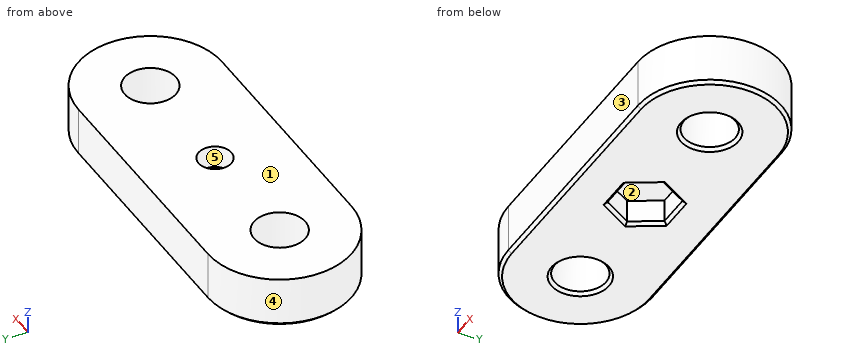
from build123d import *

# Parameters (mm, degrees)
SKETCH_R        = 2.5
SKETCH_R_2      = 1.6
PAD_DEPTH       = 5
POCKET_DEPTH    = 2.5
SKETCH002_R     = 1.6
PAD001_DEPTH    = 0.3
CHAMFER_SIZE    = 0.3
CHAMFER001_SIZE = 0.3


with BuildPart() as part:
    # Sketch → Pad (new body)
    with BuildSketch(Plane.XY):
        with BuildLine():
            ThreePointArc((-11.575, 7), (-18.575, 0), (-11.575, -7))
            Line((-11.575, -7), (11.575, -7))
            ThreePointArc((11.575, -7), (18.575, 0), (11.575, 7))
            Line((-11.575, 7), (11.575, 7))
        make_face()
        with Locations((-11.575, 0)):
            Circle(SKETCH_R, mode=Mode.SUBTRACT)
        with Locations((11.575, 0)):
            Circle(SKETCH_R, mode=Mode.SUBTRACT)
        Circle(SKETCH_R_2, mode=Mode.SUBTRACT)
    extrude(amount=PAD_DEPTH)

    # Sketch001 → Pocket (cut)
    with BuildSketch(Plane(origin=(0, 0, 0), x_dir=(1, 0, 0), z_dir=(0, 0, -1))):
        Polygon((1.602147, 2.775), (-1.602147, 2.775), (-3.204294, 0), (-1.602147, -2.775), (1.602147, -2.775), (3.204294, 0), align=None)
    extrude(amount=-POCKET_DEPTH, mode=Mode.SUBTRACT)

    # Sketch002 → Pad001 (new body)
    with BuildSketch(Plane(origin=(0, 0, 2.5), x_dir=(1, 0, 0), z_dir=(0, 0, -1))):
        Circle(SKETCH002_R)
    extrude(amount=-PAD001_DEPTH)

    # Chamfer
    chamfer_edges = [part.edges().sort_by_distance(p)[0] for p in [
        (-14.075, 0, 0),
        (9.075, 0, 0),
        (2.40322, -1.3875, 0),
        (0, -2.775, 0),
        (-2.40322, -1.3875, 0),
        (-2.40322, 1.3875, 0),
        (0, 2.775, 0),
        (2.40322, 1.3875, 0),
    ]]
    chamfer(chamfer_edges, length=CHAMFER_SIZE)

    # Chamfer001
    chamfer001_edges = [part.edges().sort_by_distance(p)[0] for p in [
        (0, 7, 0),
    ]]
    chamfer(chamfer001_edges, length=CHAMFER001_SIZE)


solid = part.part
For this review, take the finished solid that the model builds, in its own axes (mm). Face numbers are marked on the shaded views. A direction names the side the tool comes from. Round coordinates to 2 decimals unless told otherwise and drop trailing zeros. Write each loop counter-clockwise with the first axis right and the second up, starting at its lowest first coordinate (ties: lowest second). Pieces come first, ordered by that corner, then holes. Notation, with made-up numbers: (61, 14) -> (71, 14) arc R20 cw to (71, 20) -> close; hole circle Ø3 at (48, -29.75). An arc over 180 degrees is marked (long way). Use CSV: the item, a comma, the result in double quotes.
(1) Consider section A-A, the plane z = 1.85. Give the boundary of the cut face in (x, y) (3 decimals).
Computed values:
outline,"(-11.575, -7) -> (11.575, -7) arc R7 ccw to (11.575, 7) -> (-11.575, 7) arc R7 ccw to start; hole circle Ø5 at (-11.575, 0); hole (-3.204, 0) -> (-1.602, -2.775) -> (1.602, -2.775) -> (3.204, 0) -> (1.602, 2.775) -> (-1.602, 2.775) -> close; hole circle Ø5 at (11.575, 0)"
(2) Consider section B-B, the plane x = 0. Give the boundary of the cut face in (y, z) (3 decimals).
Computed values:
outline,"(-7, 0.3) -> (-6.7, 0) -> (-3.075, 0) -> (-2.775, 0.3) -> (-2.775, 2.5) -> (2.775, 2.5) -> (2.775, 0.3) -> (3.075, 0) -> (6.7, 0) -> (7, 0.3) -> (7, 5) -> (1.6, 5) -> (1.6, 2.8) -> (-1.6, 2.8) -> (-1.6, 5) -> (-7, 5) -> close"
(3) To check wall thickness, follow L1, parallel to Y at x = 0, z = 3.8; L2, parallel to X at y = 1.75, z = 1.7; L3, parallel to X at y = -0.5, z = 2.65. State the ranges of each line that lie inside material, in increasing order. Write a range as [from, to].
Computed values:
L1,"[-7, -1.6], [1.6, 7]"
L2,"[-18.35, -13.36], [-9.79, -2.19], [2.19, 9.79], [13.36, 18.35]"
L3,"[-18.56, -14.02], [-9.13, 9.13], [14.02, 18.56]"
(4) For the marked faces 1 and 2, list the 3-axis set-ups (+Z, -Z, +X, -X, +Y, -Y) from which the entire face can be reached by the end or side of a thin tool; tool diameter is ignored.
Computed values:
face 1,"+Z, +X, -X, +Y, -Y"
face 2,"-Z"
(5) Clearance check with flat-ended pins moving along their axes: P1, Ø2, axis at y = 1.5, z = 1, coming from the +X side; P2, Ø1.5, axis at y = -4.5, z = 3.5, coming from the +X side; P3, Ø2.5, axis at x = 0, y = 0, coming from the +Z side. State where each tip first meets the part, or that it passes through.
Computed values:
P1,"x = 18.56"
P2,"x = 17.49"
P3,"z = 2.8"
(6) Draft analysis for pull direction X (two halves, no side actions). For the marked faces 3, 4 and 5, state which applies: +X half, -X half, draft (parallel to the pull), parting line (faces both ways), or undercut.
Computed values:
face 3,"draft"
face 4,"-X half"
face 5,"undercut"
(7) Consider section C-C, the plane z = 4.35. Give the boundary of the cut face in (x, y) (3 decimals).
Computed values:
outline,"(-11.575, -7) -> (11.575, -7) arc R7 ccw to (11.575, 7) -> (-11.575, 7) arc R7 ccw to start; hole circle Ø5 at (-11.575, 0); hole circle Ø3.2 at (0, 0); hole circle Ø5 at (11.575, 0)"
